Part print with two shaded views. Sizes in mm from the minimum x, y, z corner. A direction names the side the tool comes from. Round coordinates to 2 decimals unless told otherwise and drop trailing zeros. Write each loop counter-clockwise with the first axis right and the second up, starting at its lowest first coordinate (ties: lowest second). Pieces come first, ordered by that corner, then holes.
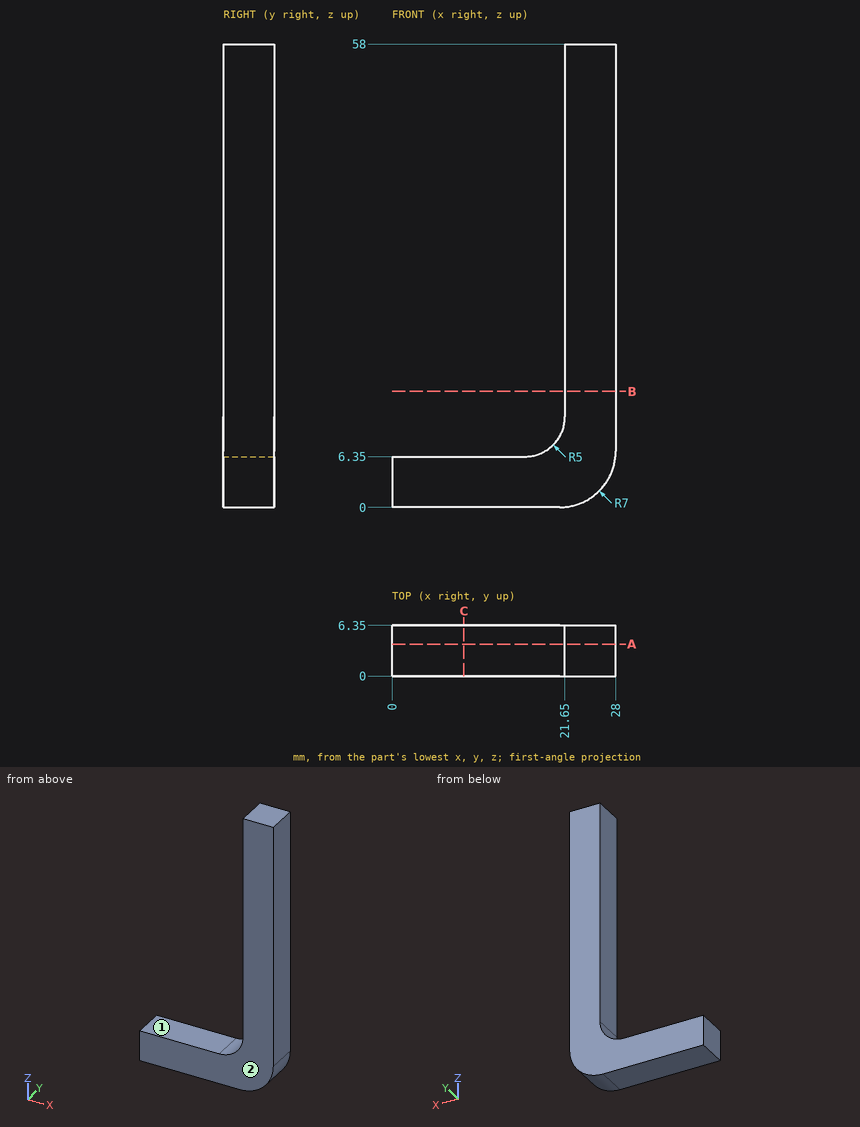
Q1. Cut at C-C on x = 9. Write the cut outline in (y, z), plus the area to 3 significant figures.
Values follow:
outline: (0, 0) - (6.35, 0) - (6.35, 6.35) - (0, 6.35) - close
area: 40.3 mm2
Q2. Drop flat-ended pins along their axis: pin 1 (3 mm diameter, centred on y = 4, z = 37, fed in from -X); pin 2 (3 mm diameter, centred on x = 4.5, z = 8, fed in from -Y). Give the stop position or say it passes through.
Values follow:
pin 1: stops at x = 21.65
pin 2: passes through
Q3. Wall check: L1, parallel to X at y = 5.75, z = 18; L2, parallel to Z at x = 8, y = 4.5; L3, parallel to Z at x = 23.75, y = 4. Give the ranges that are in metal, low to high.
Values follow:
L1: x = 21.65 to 28
L2: z = 0 to 6.35
L3: z = 0.56 to 58
Q4. Cut at A-A on y = 4. Write the cut outline in (x, z).
Values follow:
outline: (0, 0) - (21, 0) arc R7 ccw to (28, 7) - (28, 58) - (21.65, 58) - (21.65, 11.35) arc R5 cw to (16.65, 6.35) - (0, 6.35) - close
Q5. Which spindle directions (+Z, -Z, +X, -X, +Y, -Y) get a long thin tool onto all of the face, cutting with end or side? Do the marked faces 1 and 2. Say none if no direction does.
Values follow:
face 1: +Z, -X, +Y, -Y
face 2: +Z, -Z, +X, -X, -Y
Q6. Cut at B-B on z = 14.5. Write the cut outline in (x, y), plus the area to 3 significant figures.
Values follow:
outline: (21.65, 0) - (28, 0) - (28, 6.35) - (21.65, 6.35) - close
area: 40.3 mm2
